from build123d import *

# Parameters (mm, degrees)
BOSS_EXTRUDE1_DEPTH     = 33.7
FILLET1_R               = 20
FILLET2_R               = 10
CUT_EXTRUDE1_REACH      = 42.524
CUT_EXTRUDE1_END_RADIUS = 20
SKETCH18_W              = 10.7
SKETCH18_H              = 4.190618397
CUT_EXTRUDE2_REACH      = 38.996
CUT_EXTRUDE3_REACH      = 38.996
CUT_EXTRUDE4_REACH      = 41.13
CUT_EXTRUDE5_REACH      = 41.13
CUT_EXTRUDE6_REACH      = 41.13
SKETCH37_W              = 7.010527041
SKETCH37_H              = 4.046754886
CUT_EXTRUDE7_DEPTH      = 30.450302171
CUT_EXTRUDE8_DEPTH      = 10
SKETCH40_R              = 1.25
CUT_EXTRUDE9_DEPTH      = 37.995504756
SKETCH41_R              = 2.75
CUT_EXTRUDE10_DEPTH     = 5
SKETCH42_R              = 2.208277428
CUT_EXTRUDE11_DEPTH     = 3
CUT_EXTRUDE12_DEPTH     = 37.18178953
FILLET3_R               = 1
BOSS_EXTRUDE2_REACH     = 40.099
SKETCH44_R              = 2.980312175
CUT_EXTRUDE13_START     = -2.980312275
CUT_EXTRUDE13_DEPTH     = 5.96062445
CUT_EXTRUDE14_REACH     = 40.026


# Read off the part's stored shape, not the designer's step: Cut-Extrude13
with BuildPart() as part:
    # Sketch17 → Boss-Extrude1 (new body)
    with BuildSketch(Plane.XY):
        Polygon((10.53663492, 7.900076539), (10.081415975, 5.280038612), (2.74336508, 4.379039255), (-0.749806064, 3.218028635), (-0.749806064, -3.143324057), (-7.713813222, -3.143324057), (-8.111536279, 0.095870306), (-9.33663492, -4.700076539), (-9.33663492, -7.900076539), (-10.53663492, -7.900076539), (-10.53663492, -3.500076539), (-10.53663492, 6.590057575), (8.423934133, 6.030416141), align=None)
    extrude(amount=BOSS_EXTRUDE1_DEPTH)

    # Fillet1
    fillet1_edges = [part.edges().sort_by_distance(p)[0] for p in [
        (-9.33663492, -4.700076539, 16.85),
    ]]
    fillet(fillet1_edges, radius=FILLET1_R)

    # Fillet2
    fillet2_edges = [part.edges().sort_by_distance(p)[0] for p in [
        (-10.53663492, 6.590057575, 16.85),
    ]]
    fillet(fillet2_edges, radius=FILLET2_R)

    # Cut-Extrude1: up to this cylinder (the profile starts outside it)
    cut_extrude1_end = Plane(origin=(10.66336508, -7.214158247, 16.8), z_dir=(0, 0, 1)) * Cylinder(CUT_EXTRUDE1_END_RADIUS, 126.048, mode=Mode.PRIVATE)
    # Sketch18 → Cut-Extrude1 (cut, up to the surface)
    with BuildSketch(Plane.ZY.offset(10.53663492), mode=Mode.PRIVATE) as cut_extrude1_sk1:
        with Locations((16.8, -5.804767341)):
            Rectangle(SKETCH18_W, SKETCH18_H)
    cut_extrude1_tool1 = extrude(cut_extrude1_sk1.sketch, amount=-CUT_EXTRUDE1_REACH, mode=Mode.PRIVATE) - cut_extrude1_end
    add(cut_extrude1_tool1.solids().sort_by_distance((-10.536635, -5.804767, 16.8))[0], mode=Mode.SUBTRACT)

    # Cut-Extrude2: up to this plane
    cut_extrude2_end = Plane(origin=(2.74336508, 4.379039255, 33.7), z_dir=(-0.3154013115740007, 0.9489583829954822, 0))
    # Sketch32 → Cut-Extrude2 (cut, up to the surface)
    with BuildSketch(Plane.XZ.offset(3.143324057), mode=Mode.PRIVATE) as cut_extrude2_sk1:
        with BuildLine():
            Line((-0.749806064, 33.7), (-7.713813222, 33.7))
            Line((-7.713813222, 33.7), (-7.713813222, 26.689472959))
            ThreePointArc((-7.713813222, 26.689472959), (-4.231809642, 29.835), (-0.749806064, 26.689472956))
            Line((-0.749806064, 26.689472956), (-0.749806064, 33.7))
        make_face()
    cut_extrude2_tool1 = split(extrude(cut_extrude2_sk1.sketch, amount=-CUT_EXTRUDE2_REACH, mode=Mode.PRIVATE), bisect_by=cut_extrude2_end, keep=Keep.BOTH, mode=Mode.PRIVATE)
    add(cut_extrude2_tool1.solids().sort_by_distance((-4.23181, -3.143324, 31.335376))[0], mode=Mode.SUBTRACT)
    # Sketch32 → Cut-Extrude2 (cut, up to the surface)
    with BuildSketch(Plane.XZ.offset(3.143324057), mode=Mode.PRIVATE) as cut_extrude2_sk2:
        with BuildLine():
            ThreePointArc((-0.749806064, 7.010527044), (-4.231809642, 3.865), (-7.713813222, 7.010527041))
            Line((-7.713813222, 7.010527041), (-7.713813222, 0))
            Line((-7.713813222, 0), (-0.749806064, 0))
            Line((-0.749806064, 0), (-0.749806064, 7.010527044))
        make_face()
    cut_extrude2_tool2 = split(extrude(cut_extrude2_sk2.sketch, amount=-CUT_EXTRUDE2_REACH, mode=Mode.PRIVATE), bisect_by=cut_extrude2_end, keep=Keep.BOTH, mode=Mode.PRIVATE)
    add(cut_extrude2_tool2.solids().sort_by_distance((-4.23181, -3.143324, 2.364624))[0], mode=Mode.SUBTRACT)

    # Cut-Extrude3: up to this plane
    cut_extrude3_end = Plane(origin=(2.74336508, 4.379039255, 33.7), z_dir=(-0.3154013115740007, 0.9489583829954822, 0))
    # Sketch33 → Cut-Extrude3 (cut, up to the surface)
    with BuildSketch(Plane.XZ.offset(3.143324057), mode=Mode.PRIVATE) as cut_extrude3_sk1:
        with BuildLine():
            Line((-0.749806064, 26.335), (-0.749806064, 7.365))
            ThreePointArc((-0.749806064, 7.365), (-1.636617826, 9.6864927), (-3.845338986, 10.825489756))
            Line((-3.845338986, 10.825489756), (-3.845338986, 22.874510244))
            ThreePointArc((-3.845338986, 22.874510244), (-1.636617826, 24.0135073), (-0.749806064, 26.335))
        make_face()
    cut_extrude3_tool1 = split(extrude(cut_extrude3_sk1.sketch, amount=-CUT_EXTRUDE3_REACH, mode=Mode.PRIVATE), bisect_by=cut_extrude3_end, keep=Keep.BOTH, mode=Mode.PRIVATE)
    add(cut_extrude3_tool1.solids().sort_by_distance((-2.202773, -3.143324, 16.85))[0], mode=Mode.SUBTRACT)
    # Sketch33 → Cut-Extrude3 (cut, up to the surface)
    with BuildSketch(Plane.XZ.offset(3.143324057), mode=Mode.PRIVATE) as cut_extrude3_sk2:
        with BuildLine():
            Line((-7.713813222, 26.335), (-7.713813222, 7.365))
            ThreePointArc((-7.713813222, 7.365), (-6.966499846, 9.520416066), (-5.045338986, 10.750634199))
            Line((-5.045338986, 10.750634199), (-5.045338986, 22.916214753))
            Line((-5.045338986, 22.916214753), (-5.045338986, 22.949365801))
            ThreePointArc((-5.045338986, 22.949365801), (-6.966499846, 24.179583934), (-7.713813222, 26.335))
        make_face()
    cut_extrude3_tool2 = split(extrude(cut_extrude3_sk2.sketch, amount=-CUT_EXTRUDE3_REACH, mode=Mode.PRIVATE), bisect_by=cut_extrude3_end, keep=Keep.BOTH, mode=Mode.PRIVATE)
    add(cut_extrude3_tool2.solids().sort_by_distance((-6.459589, -3.143324, 16.85))[0], mode=Mode.SUBTRACT)

    # Cut-Extrude4: up to this plane
    cut_extrude4_end = Plane(origin=(-8.111536279, 0.095870306, 33.7), z_dir=(-0.9688885735577917, 0.2474973374182996, 0))
    # Sketch35 → Cut-Extrude4 (cut, up to the surface)
    with BuildSketch(Plane(origin=(-7.713813222, 0, 0), x_dir=(0, 0, -1), z_dir=(1, 0, 0)), mode=Mode.PRIVATE) as cut_extrude4_sk1:
        Polygon((-33.7, 0.903430829), (-26.689472959, 0.903430829), (-26.51223648, -3.143324057), (-33.7, -3.143324057), align=None)
    cut_extrude4_tool1 = split(extrude(cut_extrude4_sk1.sketch, amount=-CUT_EXTRUDE4_REACH, mode=Mode.PRIVATE), bisect_by=cut_extrude4_end, keep=Keep.BOTH, mode=Mode.PRIVATE)
    add(cut_extrude4_tool1.solids().sort_by_distance((-7.713813, -1.128366, 30.150243))[0], mode=Mode.SUBTRACT)

    # Cut-Extrude5: up to this plane
    cut_extrude5_end = Plane(origin=(-8.111536279, 0.095870306, 33.7), z_dir=(-0.9688885735577917, 0.2474973374182996, 0))
    # Sketch36 → Cut-Extrude5 (cut, up to the surface)
    with BuildSketch(Plane(origin=(-7.713813222, 0, 0), x_dir=(0, 0, -1), z_dir=(1, 0, 0)), mode=Mode.PRIVATE) as cut_extrude5_sk1:
        Polygon((-7.385460395, -3.179256499), (-26.335, -3.143324057), (-26.335, 0.903430829), (-7.365, 0.903430829), align=None)
    cut_extrude5_tool1 = split(extrude(cut_extrude5_sk1.sketch, amount=-CUT_EXTRUDE5_REACH, mode=Mode.PRIVATE), bisect_by=cut_extrude5_end, keep=Keep.BOTH, mode=Mode.PRIVATE)
    add(cut_extrude5_tool1.solids().sort_by_distance((-7.713813, -1.128579, 16.84114))[0], mode=Mode.SUBTRACT)

    # Cut-Extrude6: up to this plane
    cut_extrude6_end = Plane(origin=(-8.111536279, 0.095870306, 33.7), z_dir=(-0.9688885735577917, 0.2474973374182996, 0))
    # Sketch37 → Cut-Extrude6 (cut, up to the surface)
    with BuildSketch(Plane(origin=(-7.713813222, 0, 0), x_dir=(0, 0, -1), z_dir=(1, 0, 0)), mode=Mode.PRIVATE) as cut_extrude6_sk1:
        with Locations((-3.505263521, -1.119946614)):
            Rectangle(SKETCH37_W, SKETCH37_H)
    cut_extrude6_tool1 = split(extrude(cut_extrude6_sk1.sketch, amount=-CUT_EXTRUDE6_REACH, mode=Mode.PRIVATE), bisect_by=cut_extrude6_end, keep=Keep.BOTH, mode=Mode.PRIVATE)
    add(cut_extrude6_tool1.solids().sort_by_distance((-7.713813, -1.119947, 3.505264))[0], mode=Mode.SUBTRACT)

    # Sketch38 → Cut-Extrude7 (cut, through all)
    with BuildSketch(Plane(origin=(0, 0.036931473, 7.369342463), x_dir=(1, 0, 0), z_dir=(0, 0.005011438902896351, 0.999987442661218))):
        Polygon((-7.713813222, 0.866510236), (-7.905249318, 0.866510236), (-8.111536279, 0.058939572), (-7.713813222, -3.180295466), align=None)
    extrude(amount=-CUT_EXTRUDE7_DEPTH, mode=Mode.SUBTRACT)

    # Sketch39 → Cut-Extrude8 (cut)
    with BuildSketch(Plane(origin=(0, 0, 26.335), x_dir=(-1, 0, 0), z_dir=(0, 0, -1))):
        Polygon((7.905249318, 0.903430829), (7.713813222, 0.903430829), (7.713813222, -3.143324057), (8.111536279, 0.095870306), align=None)
    extrude(amount=-CUT_EXTRUDE8_DEPTH, mode=Mode.SUBTRACT)

    # Sketch40 → Cut-Extrude9 (cut, through all)
    with BuildSketch(Plane.XZ.offset(3.143324057)):
        with Locations(Location((-4.231809643, 7.365, 0), (0, 0, 270))):
            Circle(SKETCH40_R)
        with Locations(Location((-4.231809643, 26.335, 0), (0, 0, 270))):
            Circle(SKETCH40_R)
    extrude(amount=-CUT_EXTRUDE9_DEPTH, mode=Mode.SUBTRACT)

    # Sketch41 → Cut-Extrude10 (cut)
    with BuildSketch(Plane.XZ.offset(3.143324057)):
        with Locations(Location((-4.231809643, 26.335, 0), (0, 0, 270))):
            Circle(SKETCH41_R)
        with Locations(Location((-4.231809643, 7.365, 0), (0, 0, 270))):
            Circle(SKETCH41_R)
    extrude(amount=-CUT_EXTRUDE10_DEPTH, mode=Mode.SUBTRACT)

    # Sketch42 → Cut-Extrude11 (cut)
    with BuildSketch(Plane.ZX.offset(6.217374095)):
        with Locations(Location((7.365, -4.231809643, 0), (0, 0, 270))):
            Circle(SKETCH42_R)
        with Locations(Location((26.335, -4.231809643, 0), (0, 0, 270))):
            Circle(SKETCH42_R)
    extrude(amount=-CUT_EXTRUDE11_DEPTH, mode=Mode.SUBTRACT)

    # Sketch43 → Cut-Extrude12 (cut, through all)
    with BuildSketch(Plane.XY.offset(33.7)):
        Polygon((-7.905249318, 0.903430829), (-8.822914385, -1.887149193), (-9.480427728, -3.886619005), (-9.654860317, -7.900076539), (-8.364081852, -7.900076539), align=None)
    extrude(amount=-CUT_EXTRUDE12_DEPTH, mode=Mode.SUBTRACT)

    # Fillet3
    fillet3_edges = [part.edges().sort_by_distance(p)[0] for p in [
        (-9.480427728, -3.886619005, 27.925),
        (-9.480427728, -3.886619005, 5.725),
    ]]
    fillet(fillet3_edges, radius=FILLET3_R)

    # Boss-Extrude2: up to this face of the body (flat: up to its plane)
    boss_extrude2_end = Plane(part.part.faces().sort_by_distance((-1.102997501, 3.10063988, 16.85))[0])
    # Sketch44 → Boss-Extrude2 (add, up to the picked face)
    with BuildSketch(Plane(origin=(0.185171765, 6.273592006, 0), x_dir=(0.999564685295442, -0.029503218641770287, 0), z_dir=(0.029503218641770287, 0.999564685295442, 0)), mode=Mode.PRIVATE) as boss_extrude2_sk1:
        with Locations(Location((-4.641678191, 0, 0), (0, 0, 180))):
            Circle(SKETCH44_R)
    boss_extrude2_tool1 = split(extrude(boss_extrude2_sk1.sketch, amount=-BOSS_EXTRUDE2_REACH, mode=Mode.PRIVATE), bisect_by=boss_extrude2_end, keep=Keep.BOTH, mode=Mode.PRIVATE)
    add(boss_extrude2_tool1.solids().sort_by(Axis((-4.454486, 6.410536, 0), (-0.029503218641770287, -0.999564685295442, 0)))[0])

    # Cut-Extrude13 outline → Cut-Extrude13 (cut)
    with BuildSketch(Plane.XY.offset(CUT_EXTRUDE13_START)):
        with BuildLine():
            Line((-9, 3), (-7.951698739, 3))
            ThreePointArc((-7.951698739, 3), (-4.457536815, 5.489809673), (-0.241602733, 6.286188711))
            Line((-0.241602733, 6.286188711), (-1.475471034, 6.322607651))
            Line((-1.475471034, 6.322607651), (-7.433500637, 6.498465254))
            Line((-7.433500637, 6.498465254), (-9, 6.544702155))
            Line((-9, 6.544702155), (-9, 3))
        make_face()
    extrude(amount=CUT_EXTRUDE13_DEPTH, mode=Mode.SUBTRACT)

    # Cut-Extrude14: up to this plane
    cut_extrude14_end = Plane(origin=(2.74336508, 4.379039255, 33.7), z_dir=(-0.3154013115740007, 0.9489583829954822, 0))
    # Sketch47 → Cut-Extrude14 (cut, up to the surface)
    with BuildSketch(Plane.ZX.offset(6.217374095), mode=Mode.PRIVATE) as cut_extrude14_sk1:
        with BuildLine():
            Line((-2.274089727, -6.442110298), (-1.428952647, -8.002768724))
            Line((-1.428952647, -8.002768724), (0, -7.523636117))
            add(Edge.make_bspline(
                [(0, -7.523636117), (-1.334083286, -7.279775766), (-2.274089727, -6.442110298)],
                knots=[0, 0, 0, 1, 1, 1], degree=2))
        make_face()
    cut_extrude14_tool1 = split(extrude(cut_extrude14_sk1.sketch, amount=-CUT_EXTRUDE14_REACH, mode=Mode.PRIVATE), bisect_by=cut_extrude14_end, keep=Keep.BOTH, mode=Mode.PRIVATE)
    add(cut_extrude14_tool1.solids().sort_by_distance((-7.404175, 6.217374, -1.25113))[0], mode=Mode.SUBTRACT)


solid = part.part
Here's how the part is built. I have some questions about the finished solid (model axes, mm). A direction names the side the tool comes from. Round coordinates to 2 decimals unless told otherwise and drop trailing zeros. Order: outer loops, then holes, each group sorted by start corner. A loop starts at its lowest first (then second) coordinate and runs counter-clockwise, first axis right, second up. Notation, with made-up numbers: M 88,71 L 143,71 A24 cw 143,106 Z; hole C 88.5,-2 d9. An arc over 180 degrees is marked long. One line per question, with ' | ' between items.
1) Imagine slicing it at C-C, the plane x = 3.75. Write out the boundary of the cut face in (y, z).
Checked values:
outline: M 4.5,0 L 6.17,0 L 6.17,33.7 L 4.5,33.7 Z
2) Imagine slicing it at D-D, the plane z = 9. Write out the boundary of the cut face in (x, y), plus the area to 3 significant figures.
Checked values:
outline: M -10.54,-7.9 L -9.65,-7.9 L -9.49,-4.02 A1 cw -9.44,-3.76 L -7.91,0.9 L -7.71,0.9 L -7.31,1.04 L -7.31,-3.14 L -6.44,-3.14 L -6.44,1.86 L -2.02,1.86 L -2.02,-3.14 L -1.16,-3.14 L -1.16,3.08 L 2.74,4.38 L 10.08,5.28 L 10.54,7.9 L 8.42,6.03 L -0.24,6.29 A10 ccw -2.75,6.04 L -2.75,3.22 L -5.72,3.22 L -5.72,4.84 A10 ccw -10.54,-3.71 Z | area: 58.5 mm²
3) Imagine slicing it at A-A, the plane y = -1.5. Count the separate pieces of the cut face and the enclosed holes in it, plus the area to 3 significant figures.
Checked values:
separate pieces: 2 | enclosed holes: 2 | area: 97.2 mm²
4) On a 3-axis mill with a long thin cutter (end or side, diameter ignored), from which of +Z, -Z, +X, -X, +Y, -Y can I reach the whole of each face in a straight line? I mean faces 5 (the cylindrical face through (-3.319, 3.762, -2.722)), 6 (the cylindrical face through (-2.026, 4.392, 26.432)), 7 (the flat face through (-10, -6, 22.15)). Say none if no direction works.
Checked values:
face 5: -Z | face 6: +Y | face 7: +X, -X, -Y
5) I'm going to push flat-ended pins straight in: pin 1 Ø5 at (x, z) = (-4.23, 26.34) entering from -Y; pin 2 Ø5 at (y, z) = (-1.5, 23.5) entering from -X; pin 3 Ø1 at (y, z) = (1, 19) entering from -X; pin 4 Ø5 at (x, z) = (-4.23, 26.34) entering from +Y. Where does each tip first touch, or does it pass through?
Checked values:
pin 1: stops at y = 1.86 | pin 2: stops at x = -10.54 | pin 3: stops at x = -9.61 | pin 4: stops at y = 6.22
6) We'd pull the mould along X, two halves only. Please class faces 1 (the flat face through (-3.845, -1, 17)), 2 (the flat face through (-10.537, -6, 28)), 3 (the flat face through (-5, 3.217, 6)), 4 (the cylindrical face through (-5.905, -0.678, 9.547)): released by +X, released by -X, zero draft, split by the parting line, or undercut.
Checked values:
face 1: released by +X | face 2: released by -X | face 3: undercut | face 4: undercut
7) Imagine slicing it at B-B, the plane z = 21. Write out the boundary of the cut face in (x, y), plus the area to 3 significant figures.
Checked values:
outline: M -10.54,-3.71 L -9.42,-3.71 L -7.91,0.9 L -7.71,0.9 L -5.05,1.79 L -5.05,-3.14 L -3.85,-3.14 L -3.85,2.19 L 2.74,4.38 L 10.08,5.28 L 10.54,7.9 L 8.42,6.03 L -0.24,6.29 A10 ccw Z | area: 57.6 mm²
8) I need wall thicknesses on line 1 (Z direction, x = -5, y = 0.5); line 2 (Z direction, x = -4.75, y = 5.25); line 3 (X direction, y = 1.25, z = 7.5). Which ranges of each line are inside material? Lowest first, please.
Checked values:
line 1: z = 3.95 to 4.72, 10.01 to 23.69, 28.98 to 29.75 | line 2: z = -2.97 to 5.22, 9.51 to 24.19, 28.48 to 33.7 | line 3: x = -9.22 to -6.98, -1.49 to -0.75
